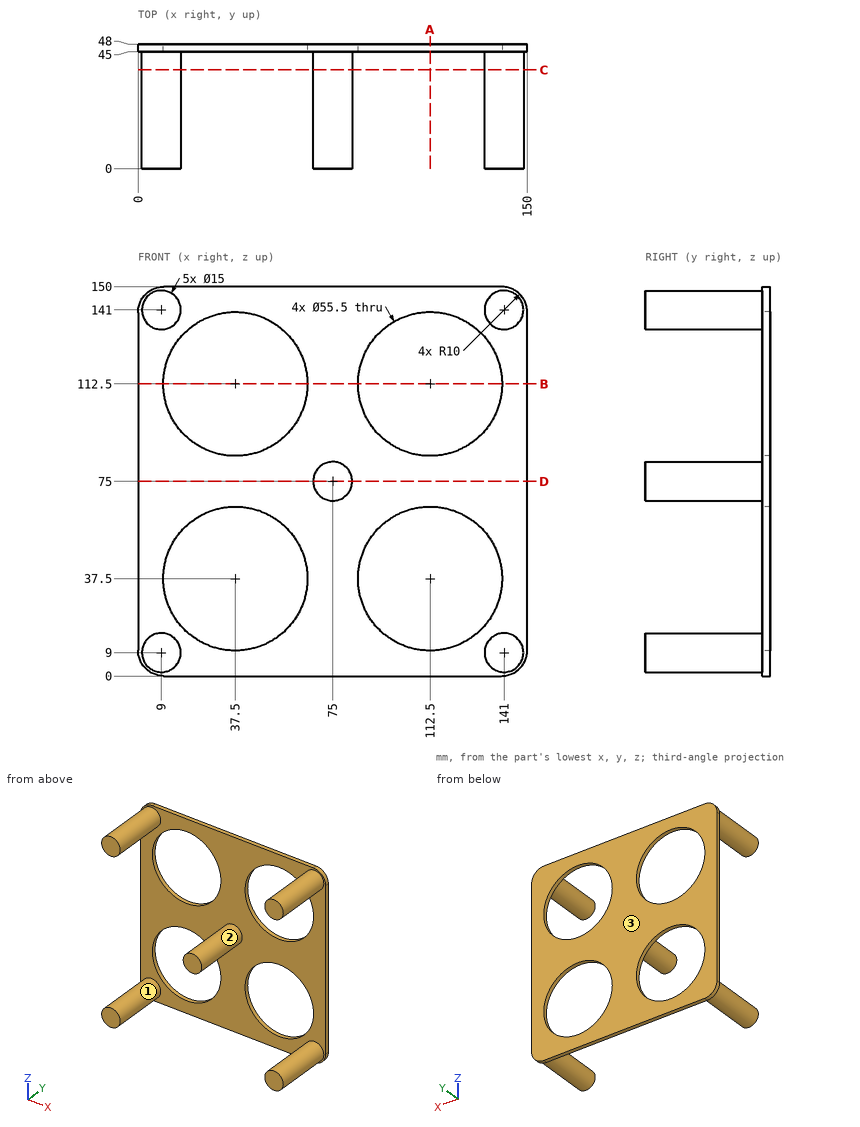
Source: three-view drawing plus pictorial views. Frame: mm from the lowest corner of the part. Give positions to 0.01 mm unless a question says otherwise; leave off trailing zeros. Order: outer loops, then holes, each group sorted by start corner. A loop starts at its lowest first (then second) coordinate and runs counter-clockwise, first axis right, second up. Notation, with made-up numbers: (-17, -18) -> (27, -18) arc R25 cw to (27, 7) -> close; hole circle Ø9 at (-5.75, 65). An arc over 180 degrees is marked (long way). Write each question's results on one line, items separated by ' | '. Start each with the question number.
Item 1: Cut plane D-D on z = 75. Return the cut outline in (x, y), then the cut area to 4 significant figures.
Item 2: Contact query for flat-ended pins moving along their axis: P1, Ø5, axis at x = 19.5, y = 20.5, coming from the +Z side; P2, Ø8, axis at x = 107.5, z = 67, coming from the -Y side. Output: stop coordinate, or through.
Item 3: Line query: line 1 (Z direction, x = 37.5, y = 47.1); line 2 (Y direction, x = 143, z = 68). Output: solid intervals per line, ascending.
Item 4: Cut plane A-A on x = 112.5. Return the cut outline in (y, z).
Item 5: Cut plane C-C on y = 38. Return the cut outline in (x, z), then the cut area to 3 significant figures.
Item 6: Cut plane B-B on z = 112.5. Return the cut outline in (x, y), then the cut area to 3 significant figures.
Item 7: Mould query, pull axis Z, two halves, no side actions, for the marked faces 1, 2 and 3. Classes: pulls with the +Z half, pulls with the -Z half, needs draft (parallel to the pull), parting line crosses it, or undercut.
Established:
1) outline: (0, 45) -> (67.5, 45) -> (67.5, 0) -> (82.5, 0) -> (82.5, 45) -> (150, 45) -> (150, 48) -> (0, 48) -> close | area: 1,125 mm^2
2) P1: through | P2: y = 45
3) line 1: 0 to 9.75, 65.25 to 84.75, 140.25 to 150 | line 2: 45 to 48
4) outline: (45, 0) -> (48, 0) -> (48, 9.75) -> (45, 9.75) -> close; (45, 65.25) -> (48, 65.25) -> (48, 84.75) -> (45, 84.75) -> close; (45, 140.25) -> (48, 140.25) -> (48, 150) -> (45, 150) -> close
5) outline: circle Ø15 at (9, 9); circle Ø15 at (9, 141); circle Ø15 at (75, 75); circle Ø15 at (141, 9); circle Ø15 at (141, 141) | area: 884 mm^2
6) outline: (0, 45) -> (9.75, 45) -> (9.75, 48) -> (0, 48) -> close; (65.25, 45) -> (84.75, 45) -> (84.75, 48) -> (65.25, 48) -> close; (140.25, 45) -> (150, 45) -> (150, 48) -> (140.25, 48) -> close | area: 117 mm^2
7) face 1: undercut | face 2: parting line crosses it | face 3: needs draft
